Design review of the part built by this model. Coordinates are the model's own, in mm. A direction names the side the tool comes from. Give positions to 0.01 mm unless a question says otherwise; leave off trailing zeros. Order: outer loops, then holes, each group sorted by start corner. A loop starts at its lowest first (then second) coordinate and runs counter-clockwise, first axis right, second up.
```python
from build123d import *

# Parameters (mm, degrees)
F0_R            = 7.95
F0_R_2          = 2
F1_DEPTH        = 2.5
F2_R            = 1.25
F3_DEPTH        = 2.5
F5_DEPTH        = 2.5
F5_COPIES_COUNT = 4


# Not quite as in the source:
# - a pattern or mirror of a feature is missing from the dataset's text; its kind, count and spacing are read off the source's solid


with BuildPart() as f1:
    # F0 (on Front) → F1 (new body)
    with BuildSketch(Plane.XZ):
        Circle(F0_R)
        Circle(F0_R_2, mode=Mode.SUBTRACT)
    extrude(amount=F1_DEPTH)

    # F2 (on face) → F3 (join)
    with BuildSketch(Plane.XZ.offset(2.5)):
        with Locations((0, 5.45)):
            Circle(F2_R)
    extrude(amount=F3_DEPTH)

    # F4 (on face) → F5 (join, through all)
    with BuildSketch(Plane.XZ.offset(2.5)):
        with BuildLine():
            ThreePointArc((-0.4960783708, 1.9375), (0, 1.5), (0.4960783708, 1.9375))
            ThreePointArc((0.4960783708, 1.9375), (0, 2), (-0.4960783708, 1.9375))
        make_face()
    f5 = extrude(amount=-F5_DEPTH)

    # F5_copies: F5 ×4 about axis
    f5_copies_axis = Axis((0, 0, 0), (0, 1, 0))
    for i in range(1, F5_COPIES_COUNT):
        add(f5.rotate(f5_copies_axis, i * 360 / F5_COPIES_COUNT))


solid = f1.part
```
1. Take a section at D-D (y = -3.35). State the section outline as (x, z) points, then the cut area to 3 significant figures.
Recorded:
outline: circle Ø2.5 at (0, 5.45)
area: 4.91 mm2
2. Take a section at A-A (z = 0). State the section outline as (x, y) points.
Recorded:
outline: (-7.95, -2.5) - (-1.5, -2.5) - (-1.5, 0) - (-7.95, 0) - close; (1.5, -2.5) - (7.95, -2.5) - (7.95, 0) - (1.5, 0) - close
3. For line 1 along X through (y, z) = (-2.3, 0.25); line 2 along Y through (x, z) = (-2.5, 6.75); line 3 along Z through (x, y) = (3, -1.25), list the stretches that pass through material, from the lowest coordinate up.
Recorded:
line 1: x = -7.95 to -1.57, 1.57 to 7.95
line 2: y = -2.5 to 0
line 3: z = -7.36 to 7.36
4. Draft analysis for pull direction Z (two halves, no side actions). For faces 1 (the face through (1.5, -1.3, 0)), 2 (the face through (-1.72, -1.23, -7.76)), 3 (the face through (1.404, -1.232, -1.425)), 4 (the face through (0, 0, -2)), state which applies: pulls with the +Z half, pulls with the -Z half, needs draft (parallel to the pull), parting line crosses it, or undercut.
Recorded:
face 1: undercut
face 2: parting line crosses it
face 3: undercut
face 4: needs draft
5. Take a section at C-C (z = 5.45). State the section outline as (x, y) points.
Recorded:
outline: (-5.79, -2.5) - (-1.25, -2.5) - (-1.25, -5) - (1.25, -5) - (1.25, -2.5) - (5.79, -2.5) - (5.79, 0) - (-5.79, 0) - close
6. Take a section at B-B (x = 0). State the section outline as (y, z) points.
Recorded:
outline: (-5, 4.2) - (-2.5, 4.2) - (-2.5, 1.5) - (0, 1.5) - (0, 7.95) - (-2.5, 7.95) - (-2.5, 6.7) - (-5, 6.7) - close; (-2.5, -7.95) - (0, -7.95) - (0, -1.5) - (-2.5, -1.5) - close
7. For pin 1 (1 mm diameter, centred on y = -1, z = -4, fed in from +X); pin 2 (4 mm diameter, centred on x = -4.5, z = -4.5, fed in from -Y), all flat-tipped, find the tip position at first contact; note any pin that passes through.
Recorded:
pin 1: stops at x = 7.14
pin 2: stops at y = -2.5
8. Machinability: for faces 5 (the face through (0, -5, 5)), 6 (the face through (-0.16, -3.73, 6.69)), which of the approach directions +Z, -Z, +X, -X, +Y, -Y give a long, thin tool a straight path to every point of the face, cutting with its end or side? Answer none if there is none.
Recorded:
face 5: +Z, -Z, +X, -X, -Y
face 6: -Y
